Verification items for the finished model (mm, model axes). A direction names the side the tool comes from. Give positions to 0.01 mm unless a question says otherwise; leave off trailing zeros. Loops run counter-clockwise (first coordinate to the right, second up) from the corner with the lowest first, then second, coordinate; pieces in that order, holes last. Notation, with made-up numbers: (64, 46.5) - (96, 46.5) arc R11 cw to (96, 54.5) - close; hole circle Ø1 at (23, -5). An arc over 180 degrees is marked (long way). Answer in a Markdown table with one row per item.
```python
from build123d import *

# Parameters (mm, degrees)
RESSALTO_EXTRUS_O1_DEPTH = 7.5
ESBO_O2_R                = 1.7
CORTE_EXTRUS_O1_DEPTH    = 60.731168581
ESBO_O3_R                = 1.7
CORTE_EXTRUS_O2_DEPTH    = 55.076912819


with BuildPart() as part:
    # Esboço1 → Ressalto-extrusão1 (new body)
    with BuildSketch(Plane.XY):
        Polygon((-23.75, 0), (-23.75, -30), (-11, -30), (-11, -48), (-5, -48), (-5, -40), (-5, -30), (0, -30), (0, -25), (-16.25, -25), (-16.25, 0), align=None)
    ressalto_extrus_o1 = extrude(amount=RESSALTO_EXTRUS_O1_DEPTH)

    # Espelhar1: Ressalto-extrusão1 across plane
    add(ressalto_extrus_o1.mirror(Plane(origin=(0, -30, 7.5), x_dir=(0, 0, 1), z_dir=(-1, 0, 0))))

    # Esboço2 → Corte-extrusão1 (cut, through all)
    with BuildSketch(Plane(origin=(11, 0, 0), x_dir=(0, 0, -1), z_dir=(1, 0, 0))):
        with Locations(Location((-3.75, -42, 0), (0, 0, 90))):
            Circle(ESBO_O2_R)
    extrude(amount=-CORTE_EXTRUS_O1_DEPTH, mode=Mode.SUBTRACT)

    # Esboço3 → Corte-extrusão2 (cut, through all)
    with BuildSketch(Plane(origin=(0, 0, 0), x_dir=(1, 0, 0), z_dir=(0, 1, 0))):
        with Locations(Location((0, -3.75, 0), (0, 0, 180))):
            Circle(ESBO_O3_R)
    extrude(amount=-CORTE_EXTRUS_O2_DEPTH, mode=Mode.SUBTRACT)


solid = part.part
```
Q1. Sectioned sample at A-A (x = 0). Record the cut outline in (y, z).
Completed:
| item | result |
|---|---|
| outline | (-30, 0) - (-25, 0) - (-25, 2.05) - (-30, 2.05) - close; (-30, 5.45) - (-25, 5.45) - (-25, 7.5) - (-30, 7.5) - close |
Q2. Go/stop test with flat-tipped pins: P1, Ø4.5, axis at y = -42, z = 3.75, coming from the +X side; P2, Ø2, axis at y = -42, z = 3.75, coming from the -X side; P3, Ø4, axis at y = -35.5, z = 4.5, coming from the -X side; P4, Ø2, axis at x = -15, z = 5.5, coming from the -Y side. Record where each tip stops, or that it passes through.
Completed:
| item | result |
|---|---|
| P1 | x = 11 |
| P2 | through |
| P3 | x = -11 |
| P4 | y = -30 |
Q3. Sectioned sample at D-D (y = -17). Record the cut outline in (x, z).
Completed:
| item | result |
|---|---|
| outline | (-23.75, 0) - (-16.25, 0) - (-16.25, 7.5) - (-23.75, 7.5) - close; (16.25, 0) - (23.75, 0) - (23.75, 7.5) - (16.25, 7.5) - close |
Q4. Sectioned sample at B-B (z = 3.75). Record the cut outline in (x, y), and give its area (3 significant figures).
Completed:
| item | result |
|---|---|
| outline | (-23.75, -30) - (-11, -30) - (-11, -40.3) - (-5, -40.3) - (-5, -30) - (-1.7, -30) - (-1.7, -25) - (-16.25, -25) - (-16.25, 0) - (-23.75, 0) - close; (-11, -48) - (-5, -48) - (-5, -43.7) - (-11, -43.7) - close; (1.7, -30) - (5, -30) - (5, -40.3) - (11, -40.3) - (11, -30) - (23.75, -30) - (23.75, 0) - (16.25, 0) - (16.25, -25) - (1.7, -25) - close; (5, -48) - (11, -48) - (11, -43.7) - (5, -43.7) - close |
| area | 771 mm^2 |
Q5. Thickness scan on line 1 (X direction, y = -32.5, z = 4.5); line 2 (Z direction, x = 0, y = -28.2); line 3 (X direction, y = -24, z = 3.5). Record the ranges inside material, lowest first.
Completed:
| item | result |
|---|---|
| line 1 | -11 to -5, 5 to 11 |
| line 2 | 0 to 2.05, 5.45 to 7.5 |
| line 3 | -23.75 to -16.25, 16.25 to 23.75 |
Q6. Draft check along X on faces 4 (the face through (11, -39, 4)), 5 (the face through (-16.25, -13, 4)), 6 (the face through (8, -48, 4)). Enter one of: +X half, -X half, draft (parallel to the pull), parting line (faces both ways), or undercut.
Completed:
| item | result |
|---|---|
| face 4 | +X half |
| face 5 | undercut |
| face 6 | draft |
Q7. Tool access check on faces 1 (the face through (1, -30, 2)), 2 (the face through (-17, -30, 4)), 3 (the face through (0, -25, 1)). Record the directions out of +Z, -Z, +X, -X, +Y, -Y that give a thin tool (end or side, any length) a straight path to the whole face; none if there is none.
Completed:
| item | result |
|---|---|
| face 1 | +Z, -Z, -Y |
| face 2 | +Z, -Z, -X, -Y |
| face 3 | +Z, -Z, +Y |
Q8. Sectioned sample at C-C (y = -42). Record the cut outline in (x, z).
Completed:
| item | result |
|---|---|
| outline | (-11, 0) - (-5, 0) - (-5, 2.05) - (-11, 2.05) - close; (-11, 5.45) - (-5, 5.45) - (-5, 7.5) - (-11, 7.5) - close; (5, 0) - (11, 0) - (11, 2.05) - (5, 2.05) - close; (5, 5.45) - (11, 5.45) - (11, 7.5) - (5, 7.5) - close |
